from build123d import *

# Parameters (mm, degrees)
SKETCH_1_W          = 38
SKETCH_1_H          = 38
SKETCH_1_R          = 1.3
EXTRUDE_1_DEPTH     = 2
SKETCH_2_W          = 38
SKETCH_2_H          = 7
SKETCH_2_R          = 1.6
EXTRUDE_2_DEPTH     = 2
SKETCH_3_R          = 5
CUT_EXTRUDE_1_DEPTH = 33.26453161
FILLET_1_R          = 1


with BuildPart() as part:
    # 草图1 → 凸台-拉伸1 (new body)
    with BuildSketch(Plane.XY):
        Rectangle(SKETCH_1_W, SKETCH_1_H)
        with BuildLine():
            Line((-14, -9.7), (-14, 9.7))
            ThreePointArc((-14, 9.7), (-10.959440841, 10.959440841), (-9.7, 14))
            Line((-9.7, 14), (9.7, 14))
            ThreePointArc((9.7, 14), (10.959440841, 10.959440841), (14, 9.7))
            Line((14, 9.7), (14, -9.7))
            ThreePointArc((14, -9.7), (10.959440841, -10.959440841), (9.7, -14))
            Line((9.7, -14), (-9.7, -14))
            ThreePointArc((-9.7, -14), (-10.959440841, -10.959440841), (-14, -9.7))
        make_face(mode=Mode.SUBTRACT)
        with Locations((14, -14)):
            Circle(SKETCH_1_R, mode=Mode.SUBTRACT)
        with Locations((14, 14)):
            Circle(SKETCH_1_R, mode=Mode.SUBTRACT)
        with Locations((-14, 14)):
            Circle(SKETCH_1_R, mode=Mode.SUBTRACT)
        with Locations((-14, -14)):
            Circle(SKETCH_1_R, mode=Mode.SUBTRACT)
    extrude(amount=EXTRUDE_1_DEPTH)

    # 草图2 → 凸台-拉伸2 (add)
    with BuildSketch(Plane.XY.offset(2)):
        with Locations((0, 22.5)):
            Rectangle(SKETCH_2_W, SKETCH_2_H)
        with Locations((-5, 23)):
            Circle(SKETCH_2_R, mode=Mode.SUBTRACT)
        with Locations((15, 23)):
            Circle(SKETCH_2_R, mode=Mode.SUBTRACT)
    extrude(amount=-EXTRUDE_2_DEPTH)

    # 草图3 → 切除-拉伸1 (cut, through all)
    with BuildSketch(Plane.XY.offset(2)):
        with Locations((0, 14)):
            Circle(SKETCH_3_R)
    extrude(amount=-CUT_EXTRUDE_1_DEPTH, mode=Mode.SUBTRACT)

    # 圆角1
    fillet_1_edges = [part.edges().sort_by_distance(p)[0] for p in [
        (19, -19, 1),
        (-19, -19, 1),
        (-14, 9.7, 1),
        (-14, -9.7, 1),
        (-9.7, -14, 1),
        (9.7, -14, 1),
        (14, -9.7, 1),
        (14, 9.7, 1),
        (9.7, 14, 1),
        (-9.7, 14, 1),
        (19, 26, 1),
        (-19, 26, 1),
        (-5, 14, 1),
        (5, 14, 1),
    ]]
    fillet(fillet_1_edges, radius=FILLET_1_R)


solid = part.part
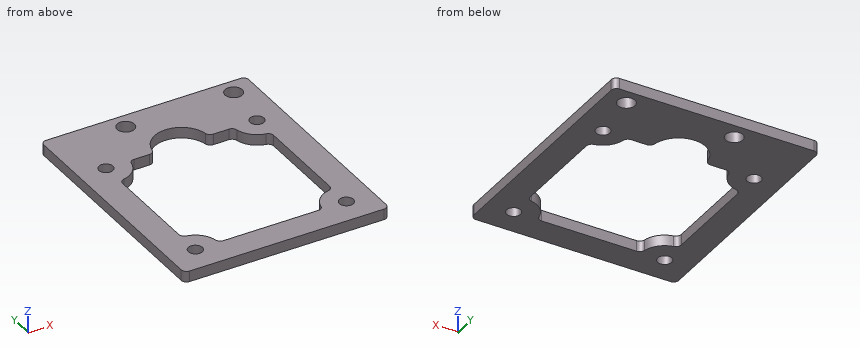
The listing builds one solid part. Answer for the finished solid, in the listing's coordinates (mm). Give positions to 0.01 mm unless a question says otherwise; leave off trailing zeros. Loops run counter-clockwise (first coordinate to the right, second up) from the corner with the lowest first, then second, coordinate; pieces in that order, holes last. Notation, with made-up numbers: (-2, 7) - (4, 7) arc R21 cw to (4, 22) - close; hole circle Ø3 at (43.25, 50.5). An arc over 180 degrees is marked (long way). Use one line per item in the form item = value.
1. Section D-D on z = 1.35 is taken. Count the separate pieces of the cut face and the enclosed holes in it, then the cut area to 3 significant figures.
Calculated:
separate_pieces = 1
enclosed_holes = 7
area = 908 mm^2
2. Section C-C on y = 0 is taken. Give the vertices of the cut face in (x, z), then the cut area to 3 significant figures.
Calculated:
outline = (-19, 0) - (-14, 0) - (-14, 2) - (-19, 2) - close; (14, 0) - (19, 0) - (19, 2) - (14, 2) - close
area = 20.0 mm^2
3. Section B-B on y = 23 is taken. Give the vertices of the cut face in (x, z), then the cut area to 3 significant figures.
Calculated:
outline = (-19, 0) - (-6.6, 0) - (-6.6, 2) - (-19, 2) - close; (-3.4, 0) - (13.4, 0) - (13.4, 2) - (-3.4, 2) - close; (16.6, 0) - (19, 0) - (19, 2) - (16.6, 2) - close
area = 63.2 mm^2
4. Find the intervals of material crossed by line 1 along Y through (x, z) = (13, 0.45); line 2 along X through (y, z) = (22, 1.4); line 3 along Y through (x, z) = (15, 1.2), in increasing order. Write a range as [from, to].
Calculated:
line_1 = [-19, -14.83], [-13.17, -9.82], [9.82, 13.17], [14.83, 26]
line_2 = [-19, -6.25], [-3.75, 13.75], [16.25, 19]
line_3 = [-19, -14.83], [-13.17, 13.17], [14.83, 21.4], [24.6, 26]
5. Section A-A on x = 4 is taken. Give the vertices of the cut face in (y, z), then the cut area to 3 significant figures.
Calculated:
outline = (-19, 0) - (-14, 0) - (-14, 2) - (-19, 2) - close; (17, 0) - (26, 0) - (26, 2) - (17, 2) - close
area = 28.0 mm^2
